from build123d import *

# Parameters (mm, degrees)
F0_W     = 22.352
F0_H     = 22.352
F1_DEPTH = 990.6


with BuildPart() as f1:
    # F0 (on Front) → F1 (new body)
    with BuildSketch(Plane.XZ):
        with BuildLine():
            ThreePointArc((0, 1.524), (0.446369, 0.446369), (1.524, 0))
            Line((1.524, 0), (23.876, 0))
            ThreePointArc((23.876, 0), (24.953631, 0.446369), (25.4, 1.524))
            Line((25.4, 1.524), (25.4, 23.876))
            ThreePointArc((25.4, 23.876), (24.953631, 24.953631), (23.876, 25.4))
            Line((23.876, 25.4), (1.524, 25.4))
            ThreePointArc((1.524, 25.4), (0.446369, 24.953631), (0, 23.876))
            Line((0, 23.876), (0, 1.524))
        make_face()
        with Locations((12.7, 12.7)):
            Rectangle(F0_W, F0_H, mode=Mode.SUBTRACT)
    extrude(amount=F1_DEPTH)


solid = f1.part
Could you check a few things on this model? Use its own coordinates, in mm. A direction names the side the tool comes from. Give positions to 0.01 mm unless a question says otherwise; leave off trailing zeros. Write each loop counter-clockwise with the first axis right and the second up, starting at its lowest first coordinate (ties: lowest second). Pieces come first, ordered by that corner, then holes. Notation, with made-up numbers: (54, 14) -> (95, 14) arc R20 ccw to (95, 21) -> close; hole circle Ø8 at (20.5, 9.25). An arc over 180 degrees is marked (long way). Answer as CSV lines item,"result". Start each with the question number.
(1) If we section it at A-A, the plane z = 6.25: Write out the boundary of the cut face in (x, y), and give its area (3 significant figures).
(2) If we section it at B-B, the plane x = 20: Write out the boundary of the cut face in (y, z), and give its area (3 significant figures).
(3) Please list where these lines run through material, in increasing order: line 1 (X direction, y = -729.5, z = 20.75); line 2 (X direction, y = -633, z = 24.5).
(4) Which directions (+Z, -Z, +X, -X, +Y, -Y) give clear straight access to the entire face, cutting with the end or side of a thin tool? Please do faces 1 (the face through (13, -488, 23.876)), 2 (the face through (13, -488, 25.4)).
(5) If we section it at C-C, the plane y = -69: Write out the boundary of the cut face in (x, z).
Answer list:
1,outline,"(0, -990.6) -> (1.52, -990.6) -> (1.52, 0) -> (0, 0) -> close; (23.88, -990.6) -> (25.4, -990.6) -> (25.4, 0) -> (23.88, 0) -> close"
1,area,"3,020 mm^2"
2,outline,"(-990.6, 0) -> (0, 0) -> (0, 1.52) -> (-990.6, 1.52) -> close; (-990.6, 23.88) -> (0, 23.88) -> (0, 25.4) -> (-990.6, 25.4) -> close"
2,area,"3,020 mm^2"
3,line 1,"0 to 1.52, 23.88 to 25.4"
3,line 2,"0.13 to 25.27"
4,face 1,"+Y, -Y"
4,face 2,"+Z, +X, -X, +Y, -Y"
5,outline,"(0, 1.52) arc R1.52 ccw to (1.52, 0) -> (23.88, 0) arc R1.52 ccw to (25.4, 1.52) -> (25.4, 23.88) arc R1.52 ccw to (23.88, 25.4) -> (1.52, 25.4) arc R1.52 ccw to (0, 23.88) -> close; hole (1.52, 1.52) -> (23.88, 1.52) -> (23.88, 23.88) -> (1.52, 23.88) -> close"
